CAD build for the part. Positions are in the model's coordinates, mm. Give positions to 0.01 mm unless a question says otherwise; leave off trailing zeros. Loops run counter-clockwise (first coordinate to the right, second up) from the corner with the lowest first, then second, coordinate; pieces in that order, holes last.
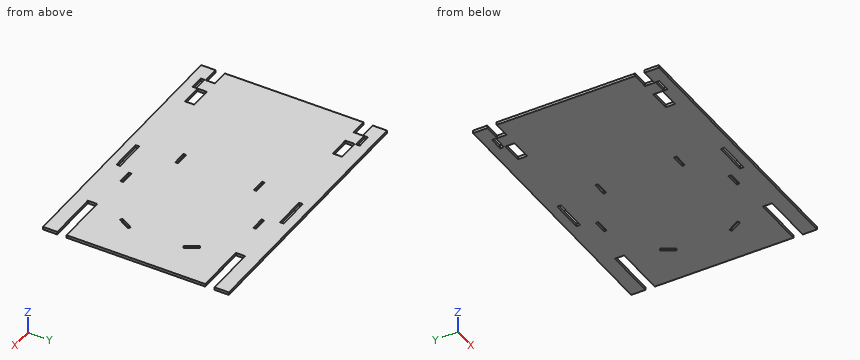
Autodesk Inventor part; units mm, degrees
ref_plane "YZ Plane" through (0, 0, 0) normal (1, 0, 0) x (0, 1, 0)
ref_plane "XZ Plane" through (0, 0, 0) normal (0, 1, 0) x (-1, 0, 0)
ref_plane "XY Plane" through (0, 0, 0) normal (0, 0, 1) x (1, 0, 0)
sketch "Sketch1" plane through (0, 0, 0) normal (0, 0, 1) x (1, 0, 0)
  line L0 (0.909, 16.8369) -> (0.909, 1.3644)
  line L1 (0.909, 1.3644) -> (290.909, 1.3644)
  line L2 (0.909, 175.8919) -> (0.909, 26.8369)
  line L3 (290.909, 185.9921) -> (290.909, 201.3644)
  line L4 (290.909, 201.3644) -> (0.909, 201.3644)
  line L5 (0.909, 201.3644) -> (0.909, 185.8919)
  line L6 (290.909, 26.7367) -> (290.909, 175.9921)
  line L7 (290.909, 1.3644) -> (290.909, 16.7367)
  line L8 (290.909, 26.7367) -> (290.909, 175.9921)
  line L9 (0.909, 16.8369) -> (0.909, 1.3644)
  line L10 (0.909, 1.3644) -> (290.909, 1.3644)
  line L11 (290.909, 1.3644) -> (290.909, 16.7367)
  line L12 (0.909, 175.8919) -> (0.909, 26.8369)
  line L13 (138.409, 187.457) -> (138.409, 191.457)
  line L14 (138.409, 191.457) -> (173.409, 191.457)
  line L15 (173.409, 191.457) -> (173.409, 187.457)
  line L16 (173.409, 187.457) -> (138.409, 187.457)
  line L17 (173.409, 11.457) -> (138.409, 11.457)
  line L18 (138.409, 11.457) -> (138.409, 15.457)
  line L19 (138.409, 15.457) -> (173.409, 15.457)
  line L20 (173.409, 15.457) -> (173.409, 11.457)
  line L21 (290.909, 175.9921) -> (234.909, 175.9921)
  line L22 (234.909, 175.9921) -> (234.909, 185.9921)
  line L23 (234.909, 185.9921) -> (290.909, 185.9921)
  line L24 (56.909, 185.8919) -> (56.909, 175.8919)
  line L25 (178.409, 173.457) -> (193.409, 173.457)
  line L26 (193.409, 173.457) -> (193.409, 170.457)
  line L27 (193.409, 170.457) -> (178.409, 170.457)
  line L28 (178.409, 170.457) -> (178.409, 173.457)
  line L29 (126.4391, 143.4522) -> (129.0372, 141.9522)
  line L30 (252.8788, 70.4522) -> (245.3788, 57.4618)
  line L31 (245.3788, 57.4618) -> (242.7807, 58.9618)
  line L32 (242.7807, 58.9618) -> (250.2807, 71.9522)
  line L33 (250.2807, 71.9522) -> (252.8788, 70.4522)
  line L34 (129.0372, 58.9618) -> (126.4391, 57.4618)
  line L35 (242.7807, 141.9522) -> (245.3788, 143.4522)
  line L36 (245.3788, 143.4522) -> (252.8788, 130.4618)
  line L37 (252.8788, 130.4618) -> (250.2807, 128.9618)
  line L38 (250.2807, 128.9618) -> (242.7807, 141.9522)
  line L39 (193.409, 27.457) -> (178.409, 27.457)
  line L40 (178.409, 27.457) -> (178.409, 30.457)
  line L41 (178.409, 30.457) -> (193.409, 30.457)
  line L42 (193.409, 30.457) -> (193.409, 27.457)
  line L43 (290.909, 26.7367) -> (234.909, 26.7367)
  line L44 (234.909, 26.7367) -> (234.909, 16.7367)
  line L45 (234.909, 16.7367) -> (290.909, 16.7367)
  line L46 (56.909, 16.8369) -> (56.909, 26.8369)
  line L47 (18.917, 187.457) -> (33.917, 187.457)
  line L48 (33.917, 187.457) -> (33.917, 191.457)
  line L49 (33.917, 191.457) -> (18.917, 191.457)
  line L50 (18.917, 191.457) -> (18.917, 187.457)
  line L51 (33.917, 11.457) -> (33.917, 15.457)
  line L52 (33.917, 15.457) -> (18.917, 15.457)
  line L53 (18.917, 15.457) -> (18.917, 11.457)
  line L54 (18.917, 11.457) -> (33.917, 11.457)
  line L55 (18.917, 185.8919) -> (18.917, 175.8919)
  line L56 (33.917, 185.8919) -> (33.917, 175.8919)
  line L57 (0.909, 185.8919) -> (18.917, 185.8919)
  line L58 (33.917, 185.8919) -> (56.909, 185.8919)
  line L59 (56.909, 175.8919) -> (33.917, 175.8919)
  line L60 (18.917, 175.8919) -> (0.909, 175.8919)
  line L61 (18.917, 26.8369) -> (18.917, 16.8369)
  line L62 (33.917, 16.8369) -> (33.917, 26.8369)
  line L63 (56.909, 26.8369) -> (33.917, 26.8369)
  line L64 (18.917, 26.8369) -> (0.909, 26.8369)
  line L65 (0.909, 16.8369) -> (18.917, 16.8369)
  line L66 (33.917, 16.8369) -> (56.909, 16.8369)
  line L67 (127.7381, 142.7022) -> (127.7381, 144.2022)
  line L68 (127.7381, 141.2022) -> (127.7381, 142.7022)
  line L69 (127.7381, 58.2118) -> (127.7381, 59.7118)
  line L70 (127.7381, 56.7118) -> (127.7381, 58.2118)
  line L71 (127.7381, 144.2022) -> (142.7381, 144.2022)
  line L72 (142.7381, 144.2022) -> (142.7381, 141.2022)
  line L73 (142.7381, 141.2022) -> (127.7381, 141.2022)
  line L74 (127.7381, 141.2022) -> (127.7381, 144.2022)
  line L75 (127.7381, 59.7118) -> (142.7381, 59.7118)
  line L76 (142.7381, 59.7118) -> (142.7381, 56.7118)
  line L77 (142.7381, 56.7118) -> (127.7381, 56.7118)
  line L78 (127.7381, 56.7118) -> (127.7381, 59.7118)
  dimension "d266" = 1.5
  dimension "d274" = 15
  dimension "d275" = 3
  dimension "d276" = 15
  dimension "d277" = 3
extrude "Extrusion3" add sketch "Sketch1" along normal blind 3
properties part number "base_ver2_2"
1. Saw through at C-C, the plane x = 165. List the corners of the cut face in (y, z).
Responses:
outline: (1.36, 0) - (11.46, 0) - (11.46, 3) - (1.36, 3) - close; (15.46, 0) - (187.46, 0) - (187.46, 3) - (15.46, 3) - close; (191.46, 0) - (201.36, 0) - (201.36, 3) - (191.46, 3) - close
2. Probe line 1 along Y through (x, z) = (270.5, 0.35); line 2 along Y through (x, z) = (189, 0.25); line 3 along X through (y, z) = (20.5, 1.9). List the from-to ranges inside material, lowest first.
Responses:
line 1: y = 1.36 to 16.74, 26.74 to 175.99, 185.99 to 201.36
line 2: y = 1.36 to 27.46, 30.46 to 170.46, 173.46 to 201.36
line 3: x = 18.92 to 33.92, 56.91 to 234.91
3. Saw through at A-A, the plane y = 182. List the corners of the cut face in (x, z).
Responses:
outline: (18.92, 0) - (33.92, 0) - (33.92, 3) - (18.92, 3) - close; (56.91, 0) - (234.91, 0) - (234.91, 3) - (56.91, 3) - close
4. Saw through at D-D, the plane z = 1.3. Count the separate pieces of the cut face and the enclosed holes in it, and give its area (3 significant figures).
Responses:
separate pieces: 1
enclosed holes: 12
area: 55,400 mm2
5. Saw through at B-B, the plane x = 262. List the corners of the cut face in (y, z), and give its area (3 significant figures).
Responses:
outline: (1.36, 0) - (16.74, 0) - (16.74, 3) - (1.36, 3) - close; (26.74, 0) - (175.99, 0) - (175.99, 3) - (26.74, 3) - close; (185.99, 0) - (201.36, 0) - (201.36, 3) - (185.99, 3) - close
area: 540 mm2
6. Drop a flat-ended pin along its axis: pin 1 (1.5 mm diameter, centred on x = 137.5, y = 69, fed in from -Z). Give the stop position or say it passes through.
Responses:
pin 1: stops at z = 0
